Part print with two shaded views. Sizes in mm from the minimum x, y, z corner. Give positions to 0.01 mm unless a question says otherwise; leave off trailing zeros. Order: outer loops, then holes, each group sorted by start corner. A loop starts at its lowest first (then second) coordinate and runs counter-clockwise, first axis right, second up. Notation, with made-up numbers: M 50.5,89 L 72.5,89 A30 cw 72.5,119 Z; hole C 31.5,18.5 d11. An arc over 180 degrees is marked long. Return JSON: item names as keys, results as strings. Group by question number.
1. Wall check: probe 1 along Y at (x, z) = (1.3, 1.2) (1 decimal); probe 2 along Y at (x, z) = (2.2, 3.2); probe 3 along Y at (x, z) = (4.5, 0.7). Give the ranges that are in metal, low to high. Write a range as [from, to].
2. Slice it at D-D on y = 31.5. List the corners of the cut face in (x, z), then the cut area to 3 significant figures.
3. Pin check, flat tip, straight feed: pin 1 (3 mm diameter, centred on x = 2.5, y = 2.5, fed in from +Z). Stop position of the tip, or through.
4. Slice it at B-B on z = 2.45. List the corners of the cut face in (x, y) (3 decimals).
5. Slice it at A-A on y = 2.5. List the corners of the cut face in (x, z) (3 decimals).
6. Two-plate mould, pull along X, no slides. Class the marked faces 1, 2, 3 and 4: released by +X, released by -X, zero draft, split by the parting line, or undercut.
7. Slice it at C-C on x = 2.95. List the corners of the cut face in (y, z).
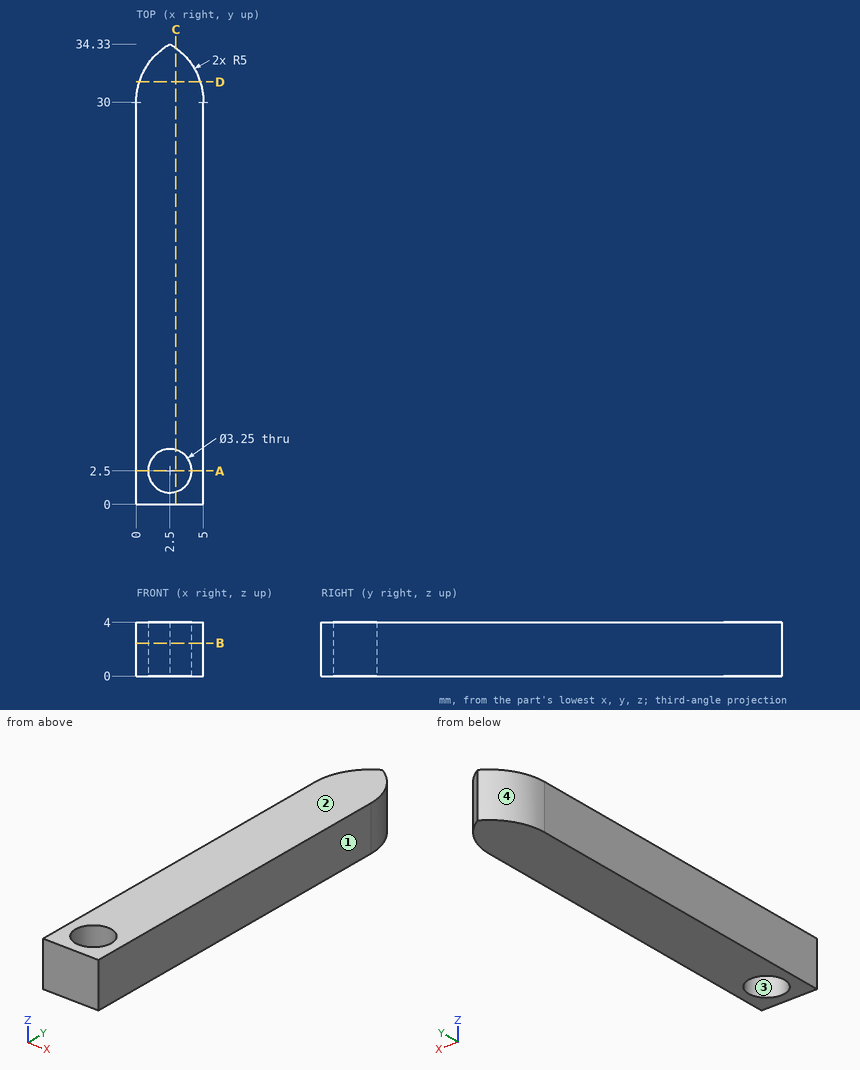
Result:
{
 "1": {"probe 1": "y = [0, 1.4], [3.6, 33.4]", "probe 2": "y = [0, 0.9], [4.1, 34.14]", "probe 3": "y = [0, 32.18]"},
 "2": {"outline": "M 0.23,0 L 4.77,0 L 4.77,4 L 0.23,4 Z", "area": "18.2 mm2"},
 "3": {"pin 1": "passes through"},
 "4": {"outline": "M 0,0 L 5,0 L 5,30 A5 ccw 2.5,34.33 A5 ccw 0,30 Z; hole C 2.5,2.5 d3.25"},
 "5": {"outline": "M 0,0 L 0.875,0 L 0.875,4 L 0,4 Z; M 4.125,0 L 5,0 L 5,4 L 4.125,4 Z"},
 "6": {"face 1": "released by +X", "face 2": "zero draft", "face 3": "undercut", "face 4": "released by -X"},
 "7": {"outline": "M 0,0 L 0.94,0 L 0.94,4 L 0,4 Z; M 4.06,0 L 34.04,0 L 34.04,4 L 4.06,4 Z"}
}
